Input: part model. Units: mm. Frame: model coordinates. Face numbers are marked on the shaded views. A direction names the side the tool comes from. Round coordinates to 2 decimals unless told otherwise and drop trailing zeros. Loops run counter-clockwise (first coordinate to the right, second up) from the corner with the lowest first, then second, coordinate; pieces in that order, holes last. Notation, with made-up numbers: (-24.5, -32.5) -> (18.5, -32.5) arc R15 cw to (18.5, -22.5) -> close; hole circle Ø10 at (15.25, 82). An arc over 180 degrees is marked (long way). One line per question, with ' | ' between items. Start each with the question number.
Q1. Material intervals for L1, parallel to Y at x = 19, z = -5; L2, parallel to Y at x = -20, z = -1.9; L3, parallel to Y at x = -19, z = -4, sorted ascending.
Q2. Mould query, pull axis Y, two halves, no side actions, for the marked faces 4, 5 and 6. Classes: pulls with the +Y half, pulls with the -Y half, needs draft (parallel to the pull), parting line crosses it, or undercut.
Q3. Cut plane C-C on y = 4.5. Return loops of the section in (x, z), and give its area (3 significant figures).
Q4. Access query for the marked faces 1, 2 and 3. Directions: +Z, -Z, +X, -X, +Y, -Y. A direction counts if a zero-diameter tool reaches every point of the face in a straight line with its end or side. Return the directions, or none.
Q5. Contact query for flat-ended pins moving along their axis: P1, Ø1, axis at y = 14, z = -3, coming from the -X side; P2, Ø2, axis at x = -24, y = -12, coming from the -Z side; P3, Ø1, axis at x = -4.5, y = 11, coming from the +Z side; P4, Ø8.5, axis at x = 9, y = 5.5, coming from the +Z side. Output: stop coordinate, or through.
Q6. Cut plane A-A on z = 1. Return loops of the section in (x, y), and give its area (3 significant figures).
Q7. Cut plane B-B on y = -3.5. Return loops of the section in (x, z), and give its area (3 significant figures).
from build123d import *

# Parameters (mm, degrees)
SKETCH1_W                                    = 75
SKETCH1_H                                    = 12
BOSS_EXTRUDE1_DEPTH                          = 17
CUT_EXTRUDE1_REACH                           = 52.973
CUT_EXTRUDE2_DEPTH                           = 1
CUT_EXTRUDE2_DEPTH_BACK                      = 1
SKETCH5_W                                    = 4
SKETCH5_H                                    = 10
SKETCH22_W                                   = 75
SKETCH22_H                                   = 34
BOSS_EXTRUDE2_DEPTH                          = 0.75
CUT_EXTRUDE3_DEPTH                           = 65.057103431
CUT_EXTRUDE3_DEPTH_BACK                      = 65.057103431
SKETCH4_R                                    = 13
CUT_EXTRUDE4_START                           = -6
CUT_EXTRUDE4_DEPTH                           = 6
SKETCH7_W                                    = 7.5
SKETCH7_H                                    = 34
CUT_EXTRUDE5_DEPTH                           = 44.102349124
CBORE_FOR_M2_HEX_SOCKET_HEAD_CAP_SCR_2_COUNT = 2
CBORE_FOR_M2_HEX_SOCKET_HEAD_CAP_SCR_2_PITCH = 50
CBORE_FOR_M2_HEX_SOCKET_HEAD_CAP_SCR_3_COUNT = 2
CBORE_FOR_M2_HEX_SOCKET_HEAD_CAP_SCR_3_PITCH = 55.461698495
CBORE_FOR_M2_HEX_SOCKET_HEAD_CAP_SCR_4_COUNT = 2
CBORE_FOR_M2_HEX_SOCKET_HEAD_CAP_SCR_4_PITCH = 24
CUT_EXTRUDE8_REACH                           = 38.764
FILLET1_R                                    = 2.5
CIRPATTERN1_COUNT                            = 2
FILLET1_OF_CIRPATTERN1_R                     = 2.5
MIRROR1_START                                = -6.75
MIRROR1_DEPTH                                = 6.75
CUT_EXTRUDE11_START                          = -1
CUT_EXTRUDE11_DEPTH                          = 1
M2_TAPPED_HOLE1_D                            = 1.6
M2_TAPPED_HOLE1_DEPTH                        = 3.2
M2_TAPPED_HOLE1_TIP                          = 0.480688495
M2_TAPPED_HOLE2_D                            = 1.6
M2_TAPPED_HOLE2_DEPTH                        = 6.75
M3X0_25_TAPPED_HOLE1_D                       = 2.75
M3X0_25_TAPPED_HOLE1_DEPTH                   = 6.75


# Read off the part's stored shape, not the designer's step: Mirror1
with BuildPart() as part:
    # Sketch1 → Boss-Extrude1 (new, symmetric)
    with BuildSketch(Plane(origin=(0, 0, 0), x_dir=(1, 0, 0), z_dir=(0, 1, 0))):
        Rectangle(SKETCH1_W, SKETCH1_H)
    extrude(amount=BOSS_EXTRUDE1_DEPTH, both=True)

    # Sketch2 → Cut-Extrude1 (cut, up to next)
    with BuildSketch(Plane(origin=(0, 17, 0), x_dir=(1, 0, 0), z_dir=(0, 1, 0)), mode=Mode.PRIVATE) as cut_extrude1_sk1:
        with BuildLine():
            Line((-37.5, 0), (-1.5, 0))
            ThreePointArc((-1.5, 0), (-0.5, -1), (-1.5, -2))
            Line((-1.5, -2), (-37.5, -2))
            ThreePointArc((-37.5, -2), (-38.5, -1), (-37.5, 0))
        make_face()
    cut_extrude1_tool1 = extrude(cut_extrude1_sk1.sketch, amount=-CUT_EXTRUDE1_REACH, mode=Mode.PRIVATE) & part.part
    # Sketch2 → Cut-Extrude1 (cut, up to next)
    with BuildSketch(Plane(origin=(0, 17, 0), x_dir=(1, 0, 0), z_dir=(0, 1, 0)), mode=Mode.PRIVATE) as cut_extrude1_sk2:
        with BuildLine():
            Line((37.5, -2), (1.5, -2))
            ThreePointArc((1.5, -2), (0.5, -1), (1.5, 0))
            Line((1.5, 0), (37.5, 0))
            ThreePointArc((37.5, 0), (38.5, -1), (37.5, -2))
        make_face()
    cut_extrude1_tool2 = extrude(cut_extrude1_sk2.sketch, amount=-CUT_EXTRUDE1_REACH, mode=Mode.PRIVATE) & part.part
    add(cut_extrude1_tool1.solids().sort_by_distance((-19.5, 17, 1))[0], mode=Mode.SUBTRACT)
    add(cut_extrude1_tool2.solids().sort_by_distance((19.5, 17, 1))[0], mode=Mode.SUBTRACT)

    # Sketch5 → Cut-Extrude2 (cut, two sides: drawn at the far end of the back side and taken through both)
    with BuildSketch(Plane(origin=(0, 0, 0), x_dir=(0, 0, -1), z_dir=(1, 0, 0)).offset(-CUT_EXTRUDE2_DEPTH_BACK)):
        with Locations((-1, 0)):
            Rectangle(SKETCH5_W, SKETCH5_H)
    extrude(amount=CUT_EXTRUDE2_DEPTH + CUT_EXTRUDE2_DEPTH_BACK, mode=Mode.SUBTRACT)

    # Sketch22 → Boss-Extrude2 (add)
    with BuildSketch(Plane(origin=(0, 0, -6), x_dir=(-1, 0, 0), z_dir=(0, 0, -1))):
        Rectangle(SKETCH22_W, SKETCH22_H)
    extrude(amount=BOSS_EXTRUDE2_DEPTH)

    # Sketch4 → Cut-Extrude3 (cut, two sides: drawn at the far end of the back side and taken through both)
    with BuildSketch(Plane(origin=(18.75, 0, 18.75), x_dir=(0, 1, 0), z_dir=(0.7071067811865488, 0, 0.7071067811865464)).offset(-CUT_EXTRUDE3_DEPTH_BACK)):
        with Locations(Location((0, -0.707106781, 0), (0, 0, 270))):
            Circle(SKETCH4_R)
    extrude(amount=CUT_EXTRUDE3_DEPTH + CUT_EXTRUDE3_DEPTH_BACK, mode=Mode.SUBTRACT)

    # Sketch6 → Cut-Extrude4 (cut)
    with BuildSketch(Plane.XY.offset(6).offset(CUT_EXTRUDE4_START)):
        with BuildLine():
            Line((-12.384776311, 13), (12.384776311, 13))
            ThreePointArc((12.384776311, 13), (25.384776311, 0), (12.384776311, -13))
            Line((12.384776311, -13), (-12.384776311, -13))
            ThreePointArc((-12.384776311, -13), (-25.384776311, 0), (-12.384776311, 13))
        make_face()
    extrude(amount=CUT_EXTRUDE4_DEPTH, mode=Mode.SUBTRACT)

    # Sketch7 → Cut-Extrude5 (cut, through all)
    with BuildSketch(Plane(origin=(0, 0, -6.75), x_dir=(-1, 0, 0), z_dir=(0, 0, -1))):
        with Locations((33.75, 0)):
            Rectangle(SKETCH7_W, SKETCH7_H)
        with Locations((-33.75, 0)):
            Rectangle(SKETCH7_W, SKETCH7_H)
    extrude(amount=-CUT_EXTRUDE5_DEPTH, mode=Mode.SUBTRACT)

    # Sketch13 → CBORE for M2 Hex Socket Head Cap Screw1 (revolve, cut)
    with BuildSketch(Plane(origin=(-25, 12, 2), x_dir=(0, 1, 0), z_dir=(1, 0, 0))):
        Polygon((0, 0), (0, 4), (1.2, 4), (1.2, 2.4), (2.2, 2.4), (2.2, 0), align=None)
    cbore_for_m2_hex_socket_head_cap_screw1 = revolve(axis=Axis((-25, 12, -4.35), (0, 0, 1)), mode=Mode.SUBTRACT)

    # CBORE for M2 Hex Socket Head Cap Scr 2: CBORE for M2 Hex Socket Head Cap Screw1 ×2
    with Locations(*[(i * CBORE_FOR_M2_HEX_SOCKET_HEAD_CAP_SCR_2_PITCH, 0, 0) for i in range(1, CBORE_FOR_M2_HEX_SOCKET_HEAD_CAP_SCR_2_COUNT)]):
        add(cbore_for_m2_hex_socket_head_cap_screw1, mode=Mode.SUBTRACT)

    # CBORE for M2 Hex Socket Head Cap Scr 3: CBORE for M2 Hex Socket Head Cap Screw1 ×2
    with Locations(*[Vector(0.9015230574682735, -0.43273106758477137, 0) * (i * CBORE_FOR_M2_HEX_SOCKET_HEAD_CAP_SCR_3_PITCH) for i in range(1, CBORE_FOR_M2_HEX_SOCKET_HEAD_CAP_SCR_3_COUNT)]):
        add(cbore_for_m2_hex_socket_head_cap_screw1, mode=Mode.SUBTRACT)

    # CBORE for M2 Hex Socket Head Cap Scr 4: CBORE for M2 Hex Socket Head Cap Screw1 ×2
    with Locations(*[(0, -i * CBORE_FOR_M2_HEX_SOCKET_HEAD_CAP_SCR_4_PITCH, 0) for i in range(1, CBORE_FOR_M2_HEX_SOCKET_HEAD_CAP_SCR_4_COUNT)]):
        add(cbore_for_m2_hex_socket_head_cap_screw1, mode=Mode.SUBTRACT)

    # Sketch15 → Cut-Extrude8 (cut, up to next)
    with BuildSketch(Plane(origin=(0, 0, -6.75), x_dir=(-1, 0, 0), z_dir=(0, 0, -1)), mode=Mode.PRIVATE) as cut_extrude8_sk1:
        Polygon((30, 17), (21, 17), (22.5, 15.5), (22.5, 9.5), (28.5, 9.5), (30, 8), align=None)
    cut_extrude8_tool1 = extrude(cut_extrude8_sk1.sketch, amount=-CUT_EXTRUDE8_REACH, mode=Mode.PRIVATE) & part.part
    cut_extrude8 = cut_extrude8_tool1.solids().sort_by_distance((-26.230769, 13.230769, -6.75))[0]
    add(cut_extrude8, mode=Mode.SUBTRACT)

    # Fillet1
    fillet1_edges = [part.edges().sort_by_distance(p)[0] for p in [
        (-22.5, 9.5, -3.375),
    ]]
    fillet(fillet1_edges, radius=FILLET1_R)

    # CirPattern1: Cut-Extrude8 ×2 about axis
    cirpattern1_axis = Axis((0, 0, 0), (0, 0, 1))
    for i in range(1, CIRPATTERN1_COUNT):
        add(cut_extrude8.rotate(cirpattern1_axis, i * 360 / CIRPATTERN1_COUNT), mode=Mode.SUBTRACT)

    # Fillet1 of CirPattern1
    fillet1_of_cirpattern1_edges = [part.edges().sort_by_distance(p)[0] for p in [
        (22.5, -9.5, -3.375),
    ]]
    fillet(fillet1_of_cirpattern1_edges, radius=FILLET1_OF_CIRPATTERN1_R)

    # Mirror1 outline → Mirror1 (cut)
    with BuildSketch(Plane.XY.offset(MIRROR1_START)):
        with BuildLine():
            Line((25, 9.5), (28.5, 9.5))
            Line((28.5, 9.5), (30, 8))
            Line((30, 8), (30, 17))
            Line((30, 17), (21, 17))
            Line((21, 17), (22.5, 15.5))
            Line((22.5, 15.5), (22.5, 12))
            ThreePointArc((22.5, 12), (23.232233047, 10.232233047), (25, 9.5))
        make_face()
        with BuildLine():
            Line((-22.5, -15.5), (-22.5, -12))
            ThreePointArc((-22.5, -12), (-23.232233047, -10.232233047), (-25, -9.5))
            Line((-25, -9.5), (-28.5, -9.5))
            Line((-28.5, -9.5), (-30, -8))
            Line((-30, -8), (-30, -17))
            Line((-30, -17), (-21, -17))
            Line((-21, -17), (-22.5, -15.5))
        make_face()
    extrude(amount=MIRROR1_DEPTH, mode=Mode.SUBTRACT)

    # Sketch20 → Cut-Extrude11 (cut)
    with BuildSketch(Plane.XY.offset(CUT_EXTRUDE11_START)):
        with BuildLine():
            Line((-12.384776311, -13), (12.384776311, -13))
            ThreePointArc((12.384776311, -13), (25.384776311, 0), (12.384776311, 13))
            Line((12.384776311, 13), (-12.384776311, 13))
            ThreePointArc((-12.384776311, 13), (-25.384776311, 0), (-12.384776311, -13))
        make_face()
    extrude(amount=CUT_EXTRUDE11_DEPTH, mode=Mode.SUBTRACT)

    # M2 Tapped Hole1
    with Locations(Plane.XY.offset(-1)):
        with Locations((20, 7.5), (-20, -7.5), (-20, 7.5), (20, -7.5)):
            Hole(M2_TAPPED_HOLE1_D / 2, depth=M2_TAPPED_HOLE1_DEPTH)
            with Locations((0, 0, -(M2_TAPPED_HOLE1_DEPTH + M2_TAPPED_HOLE1_TIP / 2))):  # 118° drill point
                Cone(0, M2_TAPPED_HOLE1_D / 2, M2_TAPPED_HOLE1_TIP, mode=Mode.SUBTRACT)

    # M2 Tapped Hole2
    with Locations(Plane(origin=(0, 0, -6.75), x_dir=(-1, 0, 0), z_dir=(0, 0, -1))):
        with Locations((19, 13.5), (-19, -13.5), (-19, 13.5), (19, -13.5)):
            Hole(M2_TAPPED_HOLE2_D / 2, depth=M2_TAPPED_HOLE2_DEPTH)

    # M3x0.25 Tapped Hole1
    with Locations(Plane(origin=(0, 0, -6.75), x_dir=(-1, 0, 0), z_dir=(0, 0, -1))):
        with Locations((-27.5, 0), (27.5, 0)):
            Hole(M3X0_25_TAPPED_HOLE1_D / 2, depth=M3X0_25_TAPPED_HOLE1_DEPTH)


solid = part.part
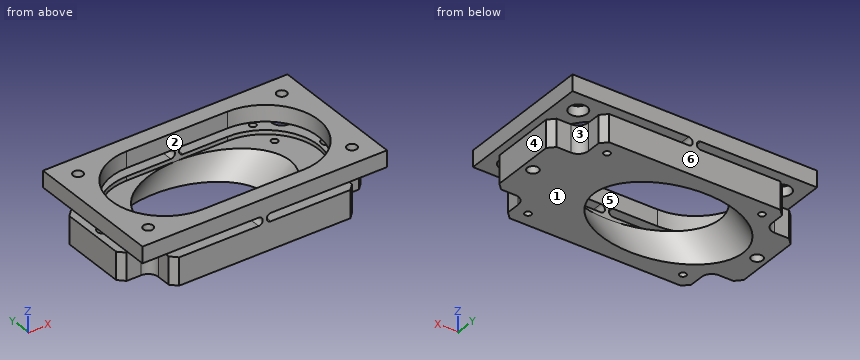
Results:
1) L1: -17 to -14.3, -12.7 to 12.7, 14.3 to 17 | L2: -17 to -8.3, -6.7 to 6.7, 8.3 to 17 | L3: -17 to -14.3, -12.7 to -6.4, 6.4 to 12.7, 14.3 to 17
2) face 4: needs draft | face 5: undercut | face 6: pulls with the +Y half
3) outline: (-30, -6.75) -> (-23, -6.75) -> (-17.25, -1) -> (-24.58, -1) -> (-24.58, 0) -> (-30, 0) -> close; (-30, 2) -> (-24.58, 2) -> (-24.58, 6) -> (-30, 6) -> close; (11.5, -6.75) -> (30, -6.75) -> (30, 0) -> (24.58, 0) -> (24.58, -1) -> (17.25, -1) -> close; (24.58, 2) -> (30, 2) -> (30, 6) -> (24.58, 6) -> close | area: 201 mm^2
4) face 1: -Z, +X, -X, +Y, -Y | face 2: +Z | face 3: -Z, +X, +Y
5) P1: x = -22.5 | P2: z = 4.4 | P3: through | P4: z = -2.85
6) outline: (-0.5, -17) -> (0.5, -17) -> (0.5, -13) -> (-0.5, -13) -> close; (-0.5, 13) -> (0.5, 13) -> (0.5, 17) -> (-0.5, 17) -> close | area: 8.00 mm^2
7) outline: (-30, -6.75) -> (-23.46, -6.75) -> (-17.71, -1) -> (-24.9, -1) -> (-24.9, 0) -> (-30, 0) -> close; (-30, 2) -> (-24.9, 2) -> (-24.9, 6) -> (-30, 6) -> close; (11.96, -6.75) -> (30, -6.75) -> (30, 0) -> (24.9, 0) -> (24.9, -1) -> (17.71, -1) -> close; (24.9, 2) -> (30, 2) -> (30, 6) -> (24.9, 6) -> close | area: 192 mm^2
